Verification items for the finished model (mm, model axes). A direction names the side the tool comes from. Coordinates: 2 decimals unless noted, no trailing zeros. Order: outer loops, then holes, each group sorted by start corner. A loop starts at its lowest first (then second) coordinate and runs counter-clockwise, first axis right, second up. Notation, with made-up numbers: M 37.25,-10 L 71.25,-10 A9 ccw 71.25,7 Z; hole C 34.25,65 d5. An arc over 180 degrees is marked long. Answer as a JSON object with one key per item and string values. Group by question number.
(1) Access from +Z, -Z, +X, -X, +Y, -Y to the whole of each face (thin tool, end or side, straight path). Record for faces 5 (the face through (0, 22, -1.35)), 6 (the face through (6, 0, -6.15)), 7 (the face through (0, -22, -1.35)).
(2) Gauge pin test, flat end, axial feed: pin 1 Ø1.8 at (x, y) = (1.5, 23.5) entering from -Z. Record the tip position at first contact, or that the pin passes through.
(3) Mould release check, pull along X, two halves, no side actions. Record for faces 1 (the face through (12.7, 0, 2)), 2 (the face through (-12.7, 0, 2)), 3 (the face through (4.197, 1.322, 0.188)), 4 (the face through (0.18, -15.86, -2.71)): released by +X, released by -X, zero draft, split by the parting line, or undercut.
(4) Cross-section at C-C (z = 3). Enter the section's corners in (x, y), plus the area to 3 significant figures.
(5) Material ranges on line 1 (Y direction, x = 0, z = 0.5); line 2 (Z direction, x = -5, y = 21.5); line 3 (X direction, y = -1, z = 0), recorded low to high.
(6) Cross-section at D-D (y = 21). Enter the section's corners in (x, z).
(7) Cross-section at A-A (y = 0). Enter the section's corners in (x, z).
(8) Cross-section at B-B (x = 0). Enter the section's corners in (y, z), plus the area to 3 significant figures.
from build123d import *

# Parameters (mm, degrees)
F1_DEPTH = 12.7
F2_R     = 4.4
F3_DEPTH = 25


with BuildPart() as f1:
    # F0 (on Right) → F1 (new body, symmetric)
    with BuildSketch(Plane.YZ):
        with BuildLine():
            Line((25.4, 6.35), (-25.4, 6.35))
            Line((-25.4, 6.35), (-25.4, -1.35))
            Line((-25.4, -1.35), (-19.2875, -1.35))
            ThreePointArc((-19.2875, -1.35), (-15.823398, -2.744449), (-14.291502, -6.15))
            Line((-14.291502, -6.15), (14.291502, -6.15))
            ThreePointArc((14.291502, -6.15), (15.823398, -2.744449), (19.2875, -1.35))
            Line((19.2875, -1.35), (25.4, -1.35))
            Line((25.4, -1.35), (25.4, 6.35))
        make_face()
    extrude(amount=F1_DEPTH, both=True)

    # F2 (on face) → F3 (cut)
    with BuildSketch(Plane.XY.offset(6.35)):
        Circle(F2_R)
    extrude(amount=-F3_DEPTH, mode=Mode.SUBTRACT)


solid = f1.part
Taken from the geometry:
{
 "1": {"face 5": "-Z, +X, -X, +Y", "face 6": "-Z, +X, -X, +Y, -Y", "face 7": "-Z, +X, -X, -Y"},
 "2": {"pin 1": "stops at z = -1.35"},
 "3": {"face 1": "released by +X", "face 2": "released by -X", "face 3": "undercut", "face 4": "zero draft"},
 "4": {"outline": "M -12.7,-25.4 L 12.7,-25.4 L 12.7,25.4 L -12.7,25.4 Z; hole C 0,0 d8.8", "area": "1,230 mm²"},
 "5": {"line 1": "y = -25.4 to -4.4, 4.4 to 25.4", "line 2": "z = -1.35 to 6.35", "line 3": "x = -12.7 to -4.28, 4.28 to 12.7"},
 "6": {"outline": "M -12.7,-1.35 L 12.7,-1.35 L 12.7,6.35 L -12.7,6.35 Z"},
 "7": {"outline": "M -12.7,-6.15 L -4.4,-6.15 L -4.4,6.35 L -12.7,6.35 Z; M 4.4,-6.15 L 12.7,-6.15 L 12.7,6.35 L 4.4,6.35 Z"},
 "8": {"outline": "M -25.4,-1.35 L -19.29,-1.35 A5 cw -14.29,-6.15 L -4.4,-6.15 L -4.4,6.35 L -25.4,6.35 Z; M 4.4,-6.15 L 14.29,-6.15 A5 cw 19.29,-1.35 L 25.4,-1.35 L 25.4,6.35 L 4.4,6.35 Z", "area": "429 mm²"}
}
